from build123d import *

# Parameters (mm, degrees)
SKETCH3_R              = 3.05
BOSS_EXTRUDE2_DEPTH    = 1.5
CUT_EXTRUDE6_START     = -1.5
CUT_EXTRUDE6_OUTLINE_R = 4.740417633
CUT_EXTRUDE6_DEPTH     = 1.5
SKETCH5_W              = 8.82084455
SKETCH5_H              = 4.027479235
CUT_EXTRUDE7_DEPTH     = 10


# Read off the part's stored shape, not the designer's step: Cut-Extrude6
with BuildPart() as part:
    # Sketch3 → Boss-Extrude2 (new body)
    with BuildSketch(Plane.XY):
        with BuildLine():
            ThreePointArc((-144.781757924, 51.155253196), (-145.537646541, 59.145084312), (-138.901541854, 63.658495821))
            Line((-138.901541854, 63.658495821), (-31.27763344, 70.484200927))
            ThreePointArc((-31.27763344, 70.484200927), (-28.219469087, 70.073170265), (-25.553222822, 68.519965104))
            Line((-25.553222822, 68.519965104), (34.035282129, 15.788374442))
            ThreePointArc((34.035282129, 15.788374442), (36.183192103, 7.089603476), (28.809941074, 1.998699544))
            Line((28.809941074, 1.998699544), (-105.054427768, 1.998699544))
            ThreePointArc((-105.054427768, 1.998699544), (-108.634306546, 2.858213585), (-111.433713401, 5.24936764))
            Line((-111.433713401, 5.24936764), (-144.781757924, 51.155253196))
        make_face()
        with Locations((-138.361865478, 55.847842692)):
            Circle(SKETCH3_R, mode=Mode.SUBTRACT)
        with Locations((-31.700427911, 60.789445495)):
            Circle(SKETCH3_R, mode=Mode.SUBTRACT)
        with Locations((28.072435844, 11.548553432)):
            Circle(SKETCH3_R, mode=Mode.SUBTRACT)
        with Locations((-20.994102553, 6.497064076)):
            Circle(SKETCH3_R, mode=Mode.SUBTRACT)
        with Locations((-104.914769783, 11.544420828)):
            Circle(SKETCH3_R, mode=Mode.SUBTRACT)
        with Locations((-59.942900407, 6.552260768)):
            Circle(SKETCH3_R, mode=Mode.SUBTRACT)
    extrude(amount=BOSS_EXTRUDE2_DEPTH)

    # Cut-Extrude6 outline → Cut-Extrude6 (cut)
    # profile 1 of 13: a face of its own
    with BuildSketch(Plane.XY.offset(1.5).offset(CUT_EXTRUDE6_START)):
        with BuildLine():
            Line((-84.445801199, 50.15994926), (-84.445801199, 31.042182393))
            ThreePointArc((-84.445801199, 31.042182393), (-83.195801199, 29.792182393), (-81.945801199, 31.042182393))
            Line((-81.945801199, 31.042182393), (-81.945801199, 40.686482216))
            Line((-81.945801199, 40.686482216), (-77.88601609, 40.686482216))
            ThreePointArc((-77.88601609, 40.686482216), (-76.63601609, 41.936482216), (-77.88601609, 43.186482216))
            Line((-77.88601609, 43.186482216), (-81.945801199, 43.186482216))
            Line((-81.945801199, 43.186482216), (-81.945801199, 50.15994926))
            ThreePointArc((-81.945801199, 50.15994926), (-81.946335576, 50.196495881), (-81.947938248, 50.233011255))
            ThreePointArc((-81.947938248, 50.233011255), (-80.383515088, 51.713053047), (-78.232158953, 51.811085227))
            ThreePointArc((-78.232158953, 51.811085227), (-76.807431812, 52.543526642), (-77.539873228, 53.968253783))
            ThreePointArc((-77.539873228, 53.968253783), (-81.355697491, 53.760646802), (-84.061279898, 51.061862018))
            ThreePointArc((-84.061279898, 51.061862018), (-84.345659533, 50.650179628), (-84.445801199, 50.15994926))
        make_face()
    # profile 2 of 13: a face of its own
    with BuildSketch(Plane.XY.offset(1.5).offset(CUT_EXTRUDE6_START)):
        with BuildLine():
            ThreePointArc((-62.332478211, 37.038133865), (-69.220904983, 43.926560636), (-76.109331754, 37.038133865))
            ThreePointArc((-76.109331754, 37.038133865), (-76.058176003, 36.667272281), (-75.908529373, 36.324108893))
            ThreePointArc((-75.908529373, 36.324108893), (-72.970069284, 31.391197022), (-67.463094766, 29.765958923))
            ThreePointArc((-67.463094766, 29.765958923), (-66.325504582, 31.119062235), (-67.678607894, 32.256652419))
            ThreePointArc((-67.678607894, 32.256652419), (-71.037890657, 33.084133952), (-73.196105391, 35.788133865))
            Line((-73.196105391, 35.788133865), (-64.262803866, 35.788133865))
            ThreePointArc((-64.262803866, 35.788133865), (-62.957767021, 35.888279837), (-62.332478211, 37.038133865))
        make_face()
        with BuildLine():
            Line((-65.265046653, 38.288133865), (-73.176763311, 38.288133865))
            ThreePointArc((-73.176763311, 38.288133865), (-69.220904982, 41.18678607), (-65.265046653, 38.288133865))
        make_face(mode=Mode.SUBTRACT)
    # profile 3 of 13: a face of its own
    with BuildSketch(Plane.XY.offset(1.5).offset(CUT_EXTRUDE6_START)):
        with BuildLine():
            Line((-88.226075166, 44.145224769), (-88.226075166, 44.594193262))
            ThreePointArc((-88.226075166, 44.594193262), (-90.027407115, 46.395525211), (-91.828739063, 44.594193262))
            Line((-91.828739063, 44.594193262), (-91.828739063, 44.145224769))
            ThreePointArc((-91.828739063, 44.145224769), (-90.027407115, 42.343892821), (-88.226075166, 44.145224769))
        make_face()
    # profile 4 of 13: a face of its own
    with BuildSketch(Plane.XY.offset(1.5).offset(CUT_EXTRUDE6_START)):
        with BuildLine():
            Line((-91.277407114, 38.985980077), (-91.277407114, 31.042182393))
            ThreePointArc((-91.277407114, 31.042182393), (-90.027407114, 29.792182393), (-88.777407114, 31.042182393))
            Line((-88.777407114, 31.042182393), (-88.777407114, 38.985980077))
            ThreePointArc((-88.777407114, 38.985980077), (-90.027407114, 40.235980077), (-91.277407114, 38.985980077))
        make_face()
    # profile 5 of 13: a face of its own
    with BuildSketch(Plane.XY.offset(1.5).offset(CUT_EXTRUDE6_START)):
        with BuildLine():
            Line((-108.731571495, 46.929777762), (-108.731571495, 31.042182393))
            ThreePointArc((-108.731571495, 31.042182393), (-108.365454972, 30.158298916), (-107.481571495, 29.792182393))
            Line((-107.481571495, 29.792182393), (-93.900874788, 29.792182393))
            ThreePointArc((-93.900874788, 29.792182393), (-92.650874788, 31.042182393), (-93.900874788, 32.292182393))
            Line((-93.900874788, 32.292182393), (-106.231571495, 32.292182393))
            Line((-106.231571495, 32.292182393), (-106.231571495, 46.929777762))
            ThreePointArc((-106.231571495, 46.929777762), (-107.481571495, 48.179777762), (-108.731571495, 46.929777762))
        make_face()
    # profile 6 of 13: a face of its own
    with BuildSketch(Plane.XY.offset(1.5).offset(CUT_EXTRUDE6_START)):
        with BuildLine():
            Line((15.808152073, 20.022138003), (-25.170273903, 57.733292534))
            ThreePointArc((-25.170273903, 57.733292534), (-28.702764122, 57.586619945), (-28.556091534, 54.054129726))
            Line((-28.556091534, 54.054129726), (12.422334441, 16.342975195))
            ThreePointArc((12.422334441, 16.342975195), (15.954824661, 16.489647783), (15.808152073, 20.022138003))
        make_face()
    # profile 7 of 13: a face of its own
    with BuildSketch(Plane.XY.offset(1.5).offset(CUT_EXTRUDE6_START)):
        with Locations((-34.929541807, 34.565020639)):
            Circle(CUT_EXTRUDE6_OUTLINE_R)
    # profile 8 of 13: a face of its own
    with BuildSketch(Plane.XY.offset(1.5).offset(CUT_EXTRUDE6_START)):
        with BuildLine():
            Line((-49.934606866, 40.291363071), (-49.934606866, 39.080866379))
            ThreePointArc((-49.934606866, 39.080866379), (-50.014724328, 38.883482639), (-50.086308054, 38.682846354))
            ThreePointArc((-50.086308054, 38.682846354), (-50.138471301, 38.116841548), (-49.934606866, 37.586255327))
            Line((-49.934606866, 37.586255327), (-49.934606866, 30.732479638))
            ThreePointArc((-49.934606866, 30.732479638), (-48.900263345, 29.698136117), (-47.865919824, 30.732479638))
            Line((-47.865919824, 30.732479638), (-47.865919824, 37.586255327))
            ThreePointArc((-47.865919824, 37.586255327), (-47.779496323, 37.734616672), (-47.714218637, 37.893421375))
            ThreePointArc((-47.714218637, 37.893421375), (-45.371600863, 39.582743631), (-43.02898309, 37.893421375))
            ThreePointArc((-43.02898309, 37.893421375), (-41.448225892, 37.102089156), (-40.656893673, 38.682846354))
            ThreePointArc((-40.656893673, 38.682846354), (-43.855198918, 41.845704884), (-48.296139271, 41.130946672))
            ThreePointArc((-48.296139271, 41.130946672), (-49.371959591, 41.211889644), (-49.934606866, 40.291363071))
        make_face()
    # profile 9 of 13: a face of its own
    with BuildSketch(Plane.XY.offset(1.5).offset(CUT_EXTRUDE6_START)):
        with BuildLine():
            Line((-5.377471622, 20.682556599), (-97.407252706, 20.682556599))
            ThreePointArc((-97.407252706, 20.682556599), (-99.907252706, 18.182556599), (-97.407252706, 15.682556599))
            Line((-97.407252706, 15.682556599), (-5.377471622, 15.682556599))
            ThreePointArc((-5.377471622, 15.682556599), (-2.877471622, 18.182556599), (-5.377471622, 20.682556599))
        make_face()
    # profile 10 of 13: a face of its own
    with BuildSketch(Plane.XY.offset(1.5).offset(CUT_EXTRUDE6_START)):
        with BuildLine():
            Line((-58.566031267, 49.850246505), (-58.566031267, 30.732479638))
            ThreePointArc((-58.566031267, 30.732479638), (-57.316031267, 29.482479638), (-56.066031267, 30.732479638))
            Line((-56.066031267, 30.732479638), (-56.066031267, 40.376779461))
            Line((-56.066031267, 40.376779461), (-52.006246159, 40.376779461))
            ThreePointArc((-52.006246159, 40.376779461), (-50.756246159, 41.626779461), (-52.006246159, 42.876779461))
            Line((-52.006246159, 42.876779461), (-56.066031267, 42.876779461))
            Line((-56.066031267, 42.876779461), (-56.066031267, 49.850246505))
            ThreePointArc((-56.066031267, 49.850246505), (-56.066565644, 49.886793126), (-56.068168316, 49.923308499))
            ThreePointArc((-56.068168316, 49.923308499), (-54.516982153, 51.397692157), (-52.379843678, 51.510052394))
            ThreePointArc((-52.379843678, 51.510052394), (-50.962005268, 52.255741402), (-51.707694277, 53.673579812))
            ThreePointArc((-51.707694277, 53.673579812), (-55.498696573, 53.440732932), (-58.181509966, 50.752159263))
            ThreePointArc((-58.181509966, 50.752159263), (-58.465889601, 50.340476873), (-58.566031267, 49.850246505))
        make_face()
    # profile 11 of 13: a face of its own
    with BuildSketch(Plane.XY.offset(1.5).offset(CUT_EXTRUDE6_START)):
        with BuildLine():
            ThreePointArc((-19.109158417, 37.228945948), (-20.160440416, 38.463049329), (-21.545976267, 37.62132764))
            ThreePointArc((-21.545976267, 37.62132764), (-28.473684687, 34.773889825), (-21.609158417, 31.777337614))
            Line((-21.609158417, 31.777337614), (-21.609158417, 28.503585324))
            ThreePointArc((-21.609158417, 28.503585324), (-23.338369309, 27.48758), (-25.305636032, 27.877834744))
            ThreePointArc((-25.305636032, 27.877834744), (-27.028433091, 27.481639975), (-26.632238322, 25.758842916))
            ThreePointArc((-26.632238322, 25.758842916), (-22.616709193, 25.083359631), (-19.299662504, 27.445128696))
            ThreePointArc((-19.299662504, 27.445128696), (-19.157728042, 27.763371797), (-19.109158417, 28.108429841))
            Line((-19.109158417, 28.108429841), (-19.109158417, 37.228945948))
        make_face()
    # profile 12 of 13: a face of its own
    with BuildSketch(Plane.XY.offset(1.5).offset(CUT_EXTRUDE6_START)):
        with BuildLine():
            Line((-106.559030622, 22.817843613), (-127.379119271, 50.951878316))
            ThreePointArc((-127.379119271, 50.951878316), (-130.875842368, 51.474303034), (-131.398267085, 47.977579937))
            Line((-131.398267085, 47.977579937), (-110.578178436, 19.843545235))
            ThreePointArc((-110.578178436, 19.843545235), (-107.08145534, 19.321120517), (-106.559030622, 22.817843613))
        make_face()
    # profile 13 of 13: a face of its own
    with BuildSketch(Plane.XY.offset(1.5).offset(CUT_EXTRUDE6_START)):
        with BuildLine():
            Line((-43.460107465, 63.853687658), (-125.288821414, 57.876383158))
            ThreePointArc((-125.288821414, 57.876383158), (-127.600047149, 55.20089524), (-124.924559231, 52.889669505))
            Line((-124.924559231, 52.889669505), (-43.095845282, 58.866974005))
            ThreePointArc((-43.095845282, 58.866974005), (-40.784619546, 61.542461923), (-43.460107465, 63.853687658))
        make_face()
    extrude(amount=CUT_EXTRUDE6_DEPTH, mode=Mode.SUBTRACT)

    # Sketch5 → Cut-Extrude7 (cut)
    with BuildSketch(Plane.XY.offset(1.5)):
        with Locations((-69.045310367, 39.34406946)):
            Rectangle(SKETCH5_W, SKETCH5_H)
    extrude(amount=-CUT_EXTRUDE7_DEPTH, mode=Mode.SUBTRACT)


solid = part.part
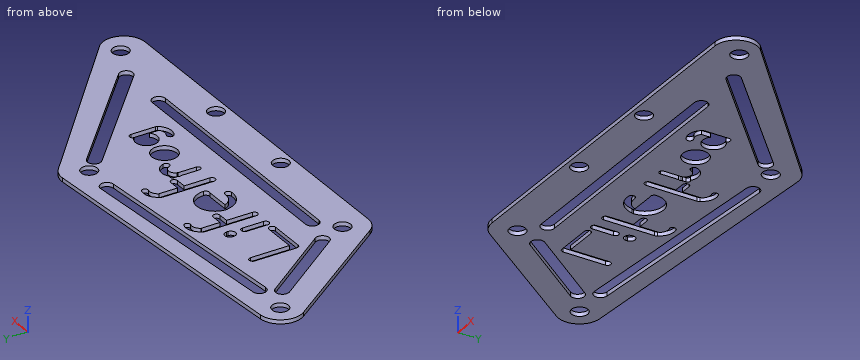
Geometry check sheet. Reference: the model listing, model coordinates, mm. Give positions to 0.01 mm unless a question says otherwise; leave off trailing zeros. Write each loop counter-clockwise with the first axis right and the second up, starting at its lowest first coordinate (ties: lowest second). Pieces come first, ordered by that corner, then holes.
1) Cross-section at B-B (z = 1.1). Count the separate pieces of the cut face and the enclosed holes in it, plus the area to 3 significant figures.
Values follow:
separate pieces: 1
enclosed holes: 19
area: 7,110 mm2
2) Thickness scan on line 1 (Y direction, x = -6.5, z = 0.5); line 2 (X direction, y = 10, z = 0.25); line 3 (Y direction, x = -117, z = 1.1). Record the ranges inside material, lowest first.
Values follow:
line 1: y = 2 to 15.68, 20.68 to 33.76, 40.55 to 51.66
line 2: x = -114.88 to -107.54, -102.28 to 25.44, 30.7 to 36.69
line 3: y = 12.91 to 28.52, 36.93 to 53.47, 58.48 to 65.05
3) Cross-section at A-A (x = -54.5). Record the boundary of the cut face in (y, z), plus the area to 3 significant figures.
Values follow:
outline: (2, 0) - (15.68, 0) - (15.68, 1.5) - (2, 1.5) - close; (20.68, 0) - (40.38, 0) - (40.38, 1.5) - (20.68, 1.5) - close; (42.88, 0) - (51.4, 0) - (51.4, 1.5) - (42.88, 1.5) - close; (53.78, 0) - (58.03, 0) - (58.03, 1.5) - (53.78, 1.5) - close; (63.05, 0) - (69.01, 0) - (69.01, 1.5) - (63.05, 1.5) - close
area: 78.2 mm2
4) Go/stop test with flat-tipped pins: pin 1 Ø0.8 at (x, z) = (-99, 0.5) entering from +Y; pin 2 Ø0.8 at (x, z) = (-70.5, 1) entering from +Y; pin 3 Ø0.8 at (y, z) = (33.5, 0.5) entering from +X; pin 4 Ø5.5 at (x, y) = (28.07, 11.55) entering from +Z. Record where each tip stops, or that it passes through.
Values follow:
pin 1: stops at y = 66.21
pin 2: stops at y = 68.02
pin 3: stops at x = 14.47
pin 4: passes through
